Here's how the part is built. I have some questions about the finished solid (model axes, mm). A direction names the side the tool comes from. Coordinates: 2 decimals unless noted, no trailing zeros. Write each loop counter-clockwise with the first axis right and the second up, starting at its lowest first coordinate (ties: lowest second). Pieces come first, ordered by that corner, then holes. Notation, with made-up numbers: (17, 51) - (71, 51) arc R19 cw to (71, 64) - close; hole circle Ø11 at (-4, -11). An arc over 180 degrees is marked (long way). Answer in a Markdown table with one row per item. Add a question column.
Item 1: I'm going to push flat-ended pins straight in: pin 1 (11 mm diameter, centred on x = 46.5, z = 103.5, fed in from -Y); pin 2 (2 mm diameter, centred on x = -7.81, z = 117.08, fed in from -Y); pin 3 (4 mm diameter, centred on x = 107.34, z = 117.08, fed in from -Y). Where does each tip first touch, or does it pass through?
Item 2: Imagine slicing it at C-C (y = 77.75). Please give me the cut outline in (x, z), plus the area to 3 significant figures.
Item 3: If I drill on probe 1 along Z at (x, y) = (93, 78.25); probe 2 along X at (y, z) = (75, 87.5); probe 3 along X at (y, z) = (77.5, 80), over which ranges is the centre line in solid material (lowest first)? Write a range as from..to.
Item 4: Imagine slicing it at A-A (z = 94). Please give me the cut outline in (x, y).
Item 5: Imagine slicing it at D-D (z = 112). Please give me the cut outline in (x, y).
Item 6: Which directions (+Z, -Z, +X, -X, +Y, -Y) give clear straight access to the entire face, cutting with the end or side of a thin tool? Please do faces 1 (the face through (107.09, 77.58, 115.13)), 2 (the face through (-8.1, 72.1, 118.3)), 3 (the face through (114.33, 73.96, 72.81)).
Item 7: We'd pull the mould along X, two halves only. Please class faces 4 (the face through (-14.89, 73.96, 124.08)), 5 (the face through (115.835, 74, 99)), 6 (the face through (-3.74, 75, 112)): +X half, -X half, draft (parallel to the pull), parting line (faces both ways), or undercut.
Item 8: Imagine slicing it at B-B (x = 8.5). Please give me the cut outline in (y, z).
from build123d import *

# Parameters (mm, degrees)
SKETCH1_W                       = 132.15
SKETCH1_H                       = 54.2
SKETCH1_W_2                     = 102
SKETCH1_H_2                     = 26.02
BOSS_EXTRUDE6_DEPTH             = 12.15
CUT_EXTRUDE9_REACH              = 13.15
SKETCH3_W                       = 105
SKETCH3_H                       = 29.02
SKETCH4_W                       = 123.15
SKETCH4_H                       = 45.2
CUT_EXTRUDE10_DEPTH             = 2.15
TAP_DRILL_FOR_M3X0_5_TAP1_D     = 2.5
TAP_DRILL_FOR_M3X0_5_TAP1_DEPTH = 4
TAP_DRILL_FOR_M3X0_5_TAP1_TIP   = 0.751075774
CUT_EXTRUDE11_DEPTH             = 9
FILLET1_R                       = 5
TAP_DRILL_FOR_M3X0_5_TAP2_D     = 2.5
TAP_DRILL_FOR_M3X0_5_TAP2_DEPTH = 5
TAP_DRILL_FOR_M3X0_5_TAP2_TIP   = 0.751075774


with BuildPart() as part:
    # Sketch1 → Boss-Extrude6 (new body)
    with BuildSketch(Plane(origin=(0, 80.115132846, 0), x_dir=(1, 0, 0), z_dir=(0, 1, 0))):
        with Locations((49.760246528, -98.484153608)):
            Rectangle(SKETCH1_W, SKETCH1_H)
        with Locations((49.760246528, -96.174153608)):
            Rectangle(SKETCH1_W_2, SKETCH1_H_2, mode=Mode.SUBTRACT)
    extrude(amount=-BOSS_EXTRUDE6_DEPTH)

    # Sketch3 → Cut-Extrude9 (cut, up to next)
    with BuildSketch(Plane(origin=(0, 79.115132846, 0), x_dir=(1, 0, 0), z_dir=(0, 1, 0)), mode=Mode.PRIVATE) as cut_extrude9_sk1:
        with Locations((49.760246528, -96.174153608)):
            Rectangle(SKETCH3_W, SKETCH3_H)
    cut_extrude9_tool1 = extrude(cut_extrude9_sk1.sketch, amount=-CUT_EXTRUDE9_REACH, mode=Mode.PRIVATE) & part.part
    add(cut_extrude9_tool1.solids().sort_by_distance((49.760247, 79.115133, 96.174154))[0], mode=Mode.SUBTRACT)

    # Sketch4 → Cut-Extrude10 (cut)
    with BuildSketch(Plane.XZ.offset(-67.965132846)):
        with Locations((49.760246528, 98.484153608)):
            Rectangle(SKETCH4_W, SKETCH4_H)
    extrude(amount=-CUT_EXTRUDE10_DEPTH, mode=Mode.SUBTRACT)

    # Tap Drill for M3x0.5 Tap1
    with Locations(Plane(origin=(0, 70.115132846, 0), x_dir=(-1, 0, 0), z_dir=(0, -1, 0))):
        with Locations((-107.335246528, -79.884153608), (-107.335246528, -117.084153608), (7.814753472, -117.084153608), (7.814753472, -79.884153608)):
            Hole(TAP_DRILL_FOR_M3X0_5_TAP1_D / 2, depth=TAP_DRILL_FOR_M3X0_5_TAP1_DEPTH)
            with Locations((0, 0, -(TAP_DRILL_FOR_M3X0_5_TAP1_DEPTH + TAP_DRILL_FOR_M3X0_5_TAP1_TIP / 2))):  # 118° drill point
                Cone(0, TAP_DRILL_FOR_M3X0_5_TAP1_D / 2, TAP_DRILL_FOR_M3X0_5_TAP1_TIP, mode=Mode.SUBTRACT)

    # Sketch8 → Cut-Extrude11 (cut)
    with BuildSketch(Plane.XZ.offset(-70.115132846)):
        Polygon((103.260246528, 77.884153608), (103.260246528, 114.884153608), (-3.739753472, 114.884153608), (-3.739753472, 109.134153608), (-9.739753472, 109.134153608), (-9.739753472, 84.134153608), (-3.739753472, 84.134153608), (-3.739753472, 77.884153608), align=None)
    extrude(amount=-CUT_EXTRUDE11_DEPTH, mode=Mode.SUBTRACT)

    # Fillet1
    fillet1_edges = [part.edges().sort_by_distance(p)[0] for p in [
        (-16.314753472, 74.040132846, 71.384153608),
        (115.835246528, 74.040132846, 71.384153608),
        (115.835246528, 74.040132846, 125.584153608),
        (-16.314753472, 74.040132846, 125.584153608),
    ]]
    fillet(fillet1_edges, radius=FILLET1_R)

    # Tap Drill for M3x0.5 Tap2
    with Locations(Plane(origin=(0, 80.115132846, 0), x_dir=(1, 0, 0), z_dir=(0, 1, 0))):
        with Locations((-8.239753472, -76.164153608), (-8.239753472, -116.184153608), (107.760246528, -116.184153608), (107.760246528, -76.164153608)):
            Hole(TAP_DRILL_FOR_M3X0_5_TAP2_D / 2, depth=TAP_DRILL_FOR_M3X0_5_TAP2_DEPTH)
            with Locations((0, 0, -(TAP_DRILL_FOR_M3X0_5_TAP2_DEPTH + TAP_DRILL_FOR_M3X0_5_TAP2_TIP / 2))):  # 118° drill point
                Cone(0, TAP_DRILL_FOR_M3X0_5_TAP2_D / 2, TAP_DRILL_FOR_M3X0_5_TAP2_TIP, mode=Mode.SUBTRACT)


solid = part.part
Here are the results:
| question | item | result |
|---|---|---|
| 1 | pin 1 | passes through |
| 1 | pin 2 | stops at y = 74.26 |
| 1 | pin 3 | stops at y = 70.12 |
| 2 | outline | (-16.31, 76.38) arc R5 ccw to (-11.31, 71.38) - (110.84, 71.38) arc R5 ccw to (115.84, 76.38) - (115.84, 120.58) arc R5 ccw to (110.84, 125.58) - (-11.31, 125.58) arc R5 ccw to (-16.31, 120.58) - close; hole (-9.74, 84.13) - (-3.74, 84.13) - (-3.74, 77.88) - (103.26, 77.88) - (103.26, 114.88) - (-3.74, 114.88) - (-3.74, 109.13) - (-9.74, 109.13) - close; hole circle Ø2.5 at (-8.24, 76.16); hole circle Ø2.5 at (-8.24, 116.18); hole circle Ø2.5 at (107.76, 76.16); hole circle Ø2.5 at (107.76, 116.18) |
| 2 | area | 3,010 mm2 |
| 3 | probe 1 | z = 71.38..77.88, 114.88..125.58 |
| 3 | probe 2 | x = -16.31..-9.74, 103.26..115.84 |
| 3 | probe 3 | x = -16.31..-3.74, 103.26..115.84 |
| 4 | outline | (-16.31, 67.97) - (-11.81, 67.97) - (-11.81, 70.12) - (-9.74, 70.12) - (-9.74, 79.12) - (-1.24, 79.12) - (-1.24, 80.12) - (-16.31, 80.12) - close; (100.76, 79.12) - (103.26, 79.12) - (103.26, 70.12) - (111.34, 70.12) - (111.34, 67.97) - (115.84, 67.97) - (115.84, 80.12) - (100.76, 80.12) - close |
| 5 | outline | (-16.31, 67.97) - (-11.81, 67.97) - (-11.81, 70.12) - (-3.74, 70.12) - (-3.74, 79.12) - (103.26, 79.12) - (103.26, 70.12) - (111.34, 70.12) - (111.34, 67.97) - (115.84, 67.97) - (115.84, 80.12) - (-16.31, 80.12) - close |
| 6 | face 1 | +Y |
| 6 | face 2 | -Y |
| 6 | face 3 | -Z, +X, +Y, -Y |
| 7 | face 4 | -X half |
| 7 | face 5 | +X half |
| 7 | face 6 | undercut |
| 8 | outline | (67.97, 71.38) - (80.12, 71.38) - (80.12, 83.16) - (79.12, 83.16) - (79.12, 77.88) - (70.12, 77.88) - (70.12, 75.88) - (67.97, 75.88) - close; (67.97, 121.08) - (70.12, 121.08) - (70.12, 114.88) - (79.12, 114.88) - (79.12, 109.18) - (80.12, 109.18) - (80.12, 125.58) - (67.97, 125.58) - close |
